For this review, take the finished solid that the model builds, in its own axes (mm). A direction names the side the tool comes from. Round coordinates to 2 decimals unless told otherwise and drop trailing zeros. Loops run counter-clockwise (first coordinate to the right, second up) from the corner with the lowest first, then second, coordinate; pieces in that order, holes last.
1) Tool access review of faces 4 (the flat face through (-0.535, 13, 200)), 5 (the flat face through (2.25, 13, -2)), 6 (the flat face through (11.634, 13.043, 189.987)), 7 (the flat face through (-0.476, 13, -22)): name each direction out of +Z, -Z, +X, -X, +Y, -Y from which nothing blocks a thin tool from reaching the whole face with its end or side.
2) Wall thickness on L1, parallel to Z at x = 9.5, y = 10.75; L2, parallel to Z at x = 2.5, y = 14.75; L3, parallel to Z at x = 6.5, y = 12.5: over which ranges is each line inside the solid? List them lowest first.
3) Insertion check: pin 1 (1.5 mm diameter, centred on y = 12, z = -2, fed in from +X); pin 2 (0.9 mm diameter, centred on x = 9, y = 12, fed in from +Z); pin 3 (2 mm diameter, centred on x = -1.5, y = 14, fed in from +Z). Each pin has a flat end and moves straight along its axis. Give the tip position at first contact, or say it passes through.
4) Take a section at A-A (z = 87). State the section outline as (x, y) points (3 decimals).
5) Mouldability with a two-part tool opening along Z and no side actions: class faces 1 (the flat face through (6, 9.752, 68)), 2 (the flat face through (6, 13, 191)), 3 (the flat face through (9.75, 13, 182)) as pulls with the +Z half, pulls with the -Z half, needs draft (parallel to the pull), parting line crosses it, or undercut.
Autodesk Inventor part; units mm, degrees
ref_plane "YZ Plane" through (0, 0, 0) normal (1, 0, 0) x (0, 1, 0)
ref_plane "XZ Plane" through (0, 0, 0) normal (0, 1, 0) x (-1, 0, 0)
ref_plane "XY Plane" through (0, 0, 0) normal (0, 0, 1) x (1, 0, 0)
sketch "Sketch1" plane through (0, 0, 0) normal (0, 0, 1) x (1, 0, 0)
  line L0 (9.75, 13) -> (7.875, 9.7524)
  line L1 (7.875, 9.7524) -> (4.125, 9.7524)
  line L2 (4.125, 9.7524) -> (2.25, 13)
  line L3 (2.25, 13) -> (4.125, 16.2476)
  line L4 (4.125, 16.2476) -> (7.875, 16.2476)
  line L5 (7.875, 16.2476) -> (9.75, 13)
  point P0 (0, 0)
  point P1 (6, 13)
  dimension "d0" = 7.5
extrude "Extrusion1" add sketch "Sketch1" along normal blind 180
sketch "Sketch2" plane through (4.125, 16.2476, 0) normal (0, 1, 0) x (1, 0, 0)
  line L0 (3.75, -180) -> (5.625, -180)
  line L1 (3.75, -180) -> (0, -180)
  line L2 (0, -180) -> (-6.6597, -195.0128)
  line L3 (-1.875, 0) -> (-1.875, -180)
  line L4 (-6.6597, -207.8247) -> (-6.6597, -195.0128)
  line L5 (3.75, -180) -> (1.875, -180)
  line L6 (9.3403, -207.8668) -> (9.3403, -194.8539)
  line L7 (9.3403, -194.8539) -> (3.75, -180)
  line L8 (9.3403, -207.8668) -> (7.3403, -207.8668)
  line L9 (7.3403, -207.8668) -> (7.3403, -195.2178)
  line L10 (-6.6597, -207.8247) -> (-4.6597, -207.8247)
  line L11 (-4.6597, -207.8247) -> (-4.6597, -195.4364)
  line L12 (2.1735, -180.0436) -> (2.158, -180)
  line L13 (1.875, -191) -> (5.7529, -191)
  line L14 (-2.6917, -191) -> (1.875, -191)
  line L15 (-4.6597, -195.4364) -> (-2.6917, -191)
  line L16 (5.7529, -191) -> (7.3403, -195.2178)
  line L17 (1.875, -180) -> (1.875, -207.8247)
  point P0 (-4.125, 0)
  dimension "d12" = 2
  dimension "d13" = 2
  dimension "d16" = 27.8247
  dimension "d17" = 11
  dimension "d21" = 12
  dimension "d31" = 2
  dimension "d32" = 2
extrude "Extrusion2" add sketch "Sketch2" against normal blind 6.5
sketch "Sketch3" plane through (-2.5347, 9.7476, 195.0128) normal (-0.9141, 0, -0.4055) x (-0.4055, 0, 0.9141)
  point P0 (-179.2885, -9.7476)
sketch "Sketch5" plane through (4.125, 16.2476, 0) normal (0, 1, 0) x (1, 0, 0)
  line L0 (-1.875, -180) -> (0, -180)
  line L1 (-1.875, -180) -> (-1.875, -184.2268)
  line L2 (0, -180) -> (-6.6597, -195.0128)
  line L3 (3.75, -180) -> (5.625, -180)
  line L4 (5.625, -180) -> (5.625, -184.982)
  line L5 (9.3403, -194.8539) -> (3.75, -180)
  point P0 (-4.125, 0)
extrude "Extrusion3" add sketch "Sketch5" against normal blind 6.5
sketch "Sketch6" plane through (13.4653, 16.2476, 207.8668) normal (1, 0, 0) x (0, 0, -1)
  line L0 (0, 0) -> (0, -3.25)
  line L1 (0, 0) -> (0, -6.5)
  line L2 (0, -3.25) -> (6, -3.25)
  circle A0 centre (6, -3.25) radius 1.5
  point P0 (207.8668, -16.2476)
  dimension "d27" = 6
  dimension "d28" = 3
extrude "Extrusion4" cut sketch "Sketch6" against normal through all
sketch "Sketch7" plane through (4.125, 9.7524, 0) normal (0, -1, 0) x (1, 0, 0)
  line L0 (0, 0) -> (-6.6005, -15.1699)
  line L1 (-6.6005, -27.9818) -> (-6.6005, -15.1699)
  line L2 (9.3995, -28.0239) -> (9.3995, -15.011)
  line L3 (9.3995, -15.011) -> (3.75, 0)
  line L4 (9.3995, -28.0239) -> (7.3995, -28.0239)
  line L5 (7.3995, -28.0239) -> (7.3995, -15.3749)
  line L6 (-6.6005, -27.9818) -> (-4.6005, -27.9818)
  line L7 (-4.6005, -27.9818) -> (-4.6005, -15.5861)
  line L8 (1.9054, -10.9999) -> (5.7124, -10.8924)
  line L9 (-2.6612, -11.129) -> (1.9054, -10.9999)
  line L10 (-4.6005, -15.5861) -> (-2.6612, -11.129)
  line L11 (5.7124, -10.8924) -> (7.3995, -15.3749)
  line L12 (1.942, 0) -> (1.942, -27.8247)
  line L13 (5.625, 0) -> (3.75, 0)
  line L14 (0, 0) -> (3.75, 0)
  line L15 (3.75, 0) -> (0, 0)
  line L16 (3.75, 0) -> (0, 0)
  point P0 (-4.125, 0)
  dimension "d34" = 2
  dimension "d35" = 2
  dimension "d36" = 11
  dimension "d37" = 12
  dimension "d38" = 2
  dimension "d39" = 2
extrude "Extrusion5" add sketch "Sketch7" against normal blind 6.5
sketch "Sketch8" plane through (1.4333, 16.2476, 191) normal (0, 1, 0) x (1, 0, 0)
  line L0 (8.3167, 191) -> (6.4417, 191)
  line L1 (8.3167, 191) -> (8.3167, 195.982)
  line L2 (12.0911, 206.011) -> (6.4417, 191)
  line L3 (2.6917, 191) -> (0.8167, 191)
  line L4 (0.8167, 191) -> (0.8167, 195.3093)
  line L5 (-3.9089, 206.1699) -> (2.6917, 191)
  point P0 (-1.4333, 191)
extrude "Extrusion6" add sketch "Sketch8" against normal blind 6.5
properties part number "Rod v1"
Response:
1. face 4: +Z, +Y, -Y
1. face 5: -X, +Y, -Y
1. face 6: +X, +Y, -Y
1. face 7: -Z, +Y, -Y
2. L1: z = -10.9 to 0, 180 to 191
2. L2: z = -11.1 to 0, 180 to 191
2. L3: z = -10.99 to 191
3. pin 1: stops at x = 9.75
3. pin 2: stops at z = 191
3. pin 3: stops at z = 207.82
4. outline: (2.25, 13) - (4.125, 9.752) - (7.875, 9.752) - (9.75, 13) - (7.875, 16.248) - (4.125, 16.248) - close
5. face 1: needs draft
5. face 2: pulls with the +Z half
5. face 3: undercut
